from build123d import *

# Parameters (mm, degrees)
SKETCH1_R           = 3.319499332
SKETCH1_R_2         = 1.86024312
SKETCH1_R_3         = 1.866358203
SKETCH1_R_4         = 1.862576991
SKETCH1_R_5         = 5
BOSS_EXTRUDE1_DEPTH = 5
SCALE1_SCALE        = 1.5


with BuildPart() as part:
    # Sketch1 → Boss-Extrude1 (new body)
    with BuildSketch(Plane.XY):
        with BuildLine():
            Line((-382.519657002, 101.671493886), (-380.669449348, 40.369064063))
            add(Edge.make_bspline(
                [(-380.669449348, 40.369064063), (-380.510075486, 35.088175777), (-376.059011151, 30.897862719), (-370.778076319, 31.057283127)],
                knots=[0.052631579, 0.052631579, 0.052631579, 0.052631579, 0.105263158, 0.105263158, 0.105263158, 0.105263158], degree=3))
            add(Edge.make_bspline(
                [(-370.778076319, 31.057283127), (-365.497188033, 31.216656989), (-361.304408032, 35.667860962), (-361.466295384, 40.948656156)],
                knots=[0.157894737, 0.157894737, 0.157894737, 0.157894737, 0.210526316, 0.210526316, 0.210526316, 0.210526316], degree=3))
            Line((-361.466295384, 40.948656156), (-361.750785175, 50.228506464))
            add(Edge.make_bspline(
                [(-361.750785175, 50.228506464), (-361.835778361, 52.39364506), (-361.180362664, 54.112685792), (-359.833970045, 55.415371618)],
                knots=[0.263157895, 0.263157895, 0.263157895, 0.263157895, 0.315789474, 0.315789474, 0.315789474, 0.315789474], degree=3))
            Line((-359.833970045, 55.415371618), (-357.334397688, 58.013854448))
            add(Edge.make_bspline(
                [(-357.334397688, 58.013854448), (-355.991914942, 59.571473289), (-355.227534814, 61.38849357), (-355.248387468, 63.55777477)],
                knots=[0.368421053, 0.368421053, 0.368421053, 0.368421053, 0.421052632, 0.421052632, 0.421052632, 0.421052632], degree=3))
            Line((-355.248387468, 63.55777477), (-355.740612523, 76.291020209))
            add(Edge.make_bspline(
                [(-355.740612523, 76.291020209), (-355.792418338, 77.812752004), (-356.366704175, 79.147601188), (-357.509736863, 80.278904258)],
                knots=[0.473684211, 0.473684211, 0.473684211, 0.473684211, 0.526315789, 0.526315789, 0.526315789, 0.526315789], degree=3))
            Line((-357.509736863, 80.278904258), (-360.989523636, 83.590706139))
            add(Edge.make_bspline(
                [(-360.989523636, 83.590706139), (-362.20931085, 84.939519155), (-362.761440742, 86.502630437), (-362.89242148, 88.200958152)],
                knots=[0.578947368, 0.578947368, 0.578947368, 0.578947368, 0.631578947, 0.631578947, 0.631578947, 0.631578947], degree=3))
            Line((-362.89242148, 88.200958152), (-363.316503038, 102.251132525))
            add(Edge.make_bspline(
                [(-363.316503038, 102.251132525), (-363.440362222, 106.355428381), (-366.156979065, 109.800631398), (-369.840498136, 111.057283127)],
                knots=[0.684210526, 0.684210526, 0.684210526, 0.684210526, 0.736842105, 0.736842105, 0.736842105, 0.736842105], degree=3))
            ThreePointArc((-369.840498136, 111.057283127), (-378.197199554, 114.445234435), (-381.585150862, 106.088533018))
            add(Edge.make_bspline(
                [(-381.585150862, 106.088533018), (-382.226602728, 104.751635805), (-382.567273667, 103.24866209), (-382.519657002, 101.671493886)],
                knots=[0.894736842, 0.894736842, 0.894736842, 0.894736842, 1, 1, 1, 1], degree=3))
        make_face()
        with Locations((-371.156901577, 41.210904817)):
            Circle(SKETCH1_R, mode=Mode.SUBTRACT)
        with Locations((-359.303466466, 75.91878991)):
            Circle(SKETCH1_R_2, mode=Mode.SUBTRACT)
        with Locations((-359.150100692, 68.896756505)):
            Circle(SKETCH1_R_3, mode=Mode.SUBTRACT)
        with Locations((-358.690863752, 62.277116942)):
            Circle(SKETCH1_R_4, mode=Mode.SUBTRACT)
        with Locations((-375.712824499, 108.572908073)):
            Circle(SKETCH1_R_5, mode=Mode.SUBTRACT)
    extrude(amount=BOSS_EXTRUDE1_DEPTH)


with BuildPart() as part_1:
    # Scale1: scaled about (-370.814087285, 71.044531915, 2.5)
    add(part.part.scale(SCALE1_SCALE).moved(Location((185.407043643, -35.522265957, -1.25))))


solid = part_1.part
The model under review builds one solid part; all positions refer to its coordinate system, in mm. Coordinates: 2 decimals unless noted, no trailing zeros. Write each loop counter-clockwise with the first axis right and the second up, starting at its lowest first coordinate (ties: lowest second). Pieces come first, ordered by that corner, then holes. Notation, with made-up numbers: (1, 16.5) - (12, 16.5) arc R13 cw to (12, 37.5) - close; hole circle Ø9 at (5, 46.5). An arc over 180 degrees is marked (long way). Answer as a JSON object with one key per item and string values. Group by question number.
1. Clearance check with flat-ended pins moving along their axes: pin 1 Ø8 at (x, y) = (-371.33, 26.29) entering from +Z; pin 2 Ø4 at (x, z) = (-364.5, 0.5) entering from -Y; pin 3 Ø2 at (x, z) = (-368, 5.5) entering from -Y (3 decimals). State where each tip first meets the part, or that it passes through.
2. To check wall thickness, follow probe 1 along Y at (x, z) = (-373, 4); probe 2 along Y at (x, z) = (-374.5, 0.25); probe 3 along Y at (x, z) = (-383, 1.25). State the ranges of each line that lie inside material, in increasing order.
3. Add section C-C (y = 73.5). Give the boundary of the cut face in (x, z), plus the area to 3 significant figures.
4. Add section A-A (y = 30). Give the boundary of the cut face in (x, z).
5. Add section D-D (y = 49). Give the boundary of the cut face in (x, z).
6. Mouldability with a two-part tool opening along X and no side actions: class faces 1 (the face through (-373, 75, 6.25)), 2 (the face through (-381.694, 136.225, 2.448)), 3 (the face through (-366.58, 27.79, 2.45)), 4 (the face through (-347.83, 69.23, 2.45)) as pulls with the +X half, pulls with the -X half, needs draft (parallel to the pull), parting line crosses it, or undercut.
7. Add section B-B (z = 3.5). Give the number of separate pieces and of enclosed holes in the cut face, plus the area to 3 significant figures.
Findings:
{
 "1": {"pin 1": "through", "pin 2": "y = 11.85", "pin 3": "y = 11.225"},
 "2": {"probe 1": "11.17 to 21.6, 30.98 to 121.9, 132.78 to 135.39", "probe 2": "11.44 to 22.46, 30.13 to 120.79, 133.88 to 136.17", "probe 3": "17.23 to 121.61, 133.07 to 135.59"},
 "3": {"outline": "(-387.06, -1.25) - (-347.99, -1.25) - (-347.99, 6.25) - (-387.06, 6.25) - close", "area": "293 mm²"},
 "4": {"outline": "(-385.75, -1.25) - (-374.65, -1.25) - (-374.65, 6.25) - (-385.75, 6.25) - close; (-368, -1.25) - (-356.92, -1.25) - (-356.92, 6.25) - (-368, 6.25) - close"},
 "5": {"outline": "(-386.32, -1.25) - (-353, -1.25) - (-353, 6.25) - (-386.32, 6.25) - close"},
 "6": {"face 1": "needs draft", "face 2": "parting line crosses it", "face 3": "undercut", "face 4": "pulls with the +X half"},
 "7": {"separate pieces": "1", "enclosed holes": "5", "area": "3,460 mm²"}
}
